Check sheet for the modelled part. Datum: model origin and axes. Units: mm. A direction names the side the tool comes from. Give positions to 0.01 mm unless a question says otherwise; leave off trailing zeros. Loops run counter-clockwise (first coordinate to the right, second up) from the corner with the lowest first, then second, coordinate; pieces in that order, holes last. Notation, with made-up numbers: M 66,-25.75 L 71,-25.75 A14 cw 71,1.25 Z; hole C 50.5,79 d9. An arc over 180 degrees is marked long. One line per question, with ' | ' between items. Start each with the question number.
Autodesk Inventor part; units mm, degrees
ref_plane "YZ Plane" through (0, 0, 0) normal (1, 0, 0) x (0, 1, 0)
ref_plane "XZ Plane" through (0, 0, 0) normal (0, 1, 0) x (-1, 0, 0)
sketch "Sketch1" plane through (0, 0, 0) normal (0, 0, 1) x (1, 0, 0)
  line L0 (0, 3.81) -> (1.746, 3.81)
  line L1 (0, 0) -> (0, 7.4896) construction
  line L2 (0, 0) -> (13.1944, 0) construction
  line L3 (0, -3.81) -> (1.746, -3.81)
  arc A0 (1.746, -3.81) -> (1.746, 3.81) centre (0, 0) ccw
  line L4 (0, 3.81) -> (0, -3.81)
  point P0 (-6.8886, 3.81)
  point P1 (6.6767, 3.81)
  point P2 (0, 4.191)
  point P3 (0, 4.191)
  point P4 (-6.8886, -3.81)
  point P5 (6.6767, -3.81)
  point P6 (0, 4.191)
  point P7 (4.191, 0)
  dimension "d1" = 0.381
  dimension "d11" = 4.191
revolve "Revolution1" add sketch "Sketch1" angle 360 about axis through (0, 0, 0) along (0, 1, 0)
sketch "Sketch2" plane through (0, 3.81, 0) normal (0, 1, 0) x (1, 0, 0)
  circle A0 centre (0, 0) radius 1.746
  dimension "d3" = 3.4919
hole "Hole1" at (0, 3.81, 0) direction (0, -1, 0) diameter 3.4798 end through all
ref_plane "Work Plane1" through (0, 0, 4.191) normal (0, 0, 1) x (1, 0, 0)
sketch "Sketch3" plane through (0, 0, 4.191) normal (0, 0, 1) x (1, 0, 0)
  line L0 (-2.159, 2.54) -> (2.159, 2.54)
  line L1 (2.159, 2.54) -> (2.159, -1.27)
  line L2 (2.159, -1.27) -> (-2.159, -1.27)
  line L3 (-2.159, -1.27) -> (-2.159, 2.54)
  line L4 (1.746, 3.81) -> (-1.746, 3.81)
  point P0 (0, 0)
  point P1 (0, 2.54)
  dimension "d13" = 4.318
  dimension "d14" = 3.81
  dimension "d15" = 1.27
extrude "Extrusion1" add sketch "Sketch3" along normal blind 10.16
ref_plane "Work Plane2" through (0, 0, 1.7399) normal (0, 0, 1) x (1, 0, 0)
extrude "Extrusion2" add sketch "Sketch3" against normal up to surface (2.4511 mm away)
sketch "Sketch4" plane through (0, -1.27, 0) normal (0, -1, 0) x (1, 0, 0)
  line L0 (2.159, 2.54) -> (2.159, 14.351)
  line L1 (2.159, 10.541) -> (-2.159, 10.541)
  line L2 (-2.159, 10.541) -> (-2.159, 14.351)
  line L3 (-2.159, 14.351) -> (2.159, 14.351)
  line L4 (2.159, 14.351) -> (2.159, 10.541) construction
  line L5 (-2.159, 14.351) -> (2.159, 14.351)
  circle A0 centre (0, 15.689) radius 0.635
  circle A1 centre (0, 15.689) radius 2.54
  circle A2 centre (-1.651, 18.401) radius 0.635
  circle A3 centre (-1.651, 18.401) radius 2.54
  point P0 (0, 0)
  point P1 (2.159, 14.351)
  point P2 (0, 14.351)
  point P3 (2.159, 14.351)
  point P4 (0.889, 18.401)
  point P5 (-2.5191, 16.014)
  point P6 (-1.3208, 17.8586)
  point P7 (0.8681, 18.0761)
  dimension "d31" = 5.08
  dimension "d22" = 3.81
  dimension "d25" = 1.27
  dimension "d27" = 5.08
  dimension "d30" = 1.27
  dimension "d32" = 1.27
  dimension "d33" = 4.318
extrude "Extrusion4" add sketch "Sketch4" along normal blind 1.27
properties part number "Left Arm" material "Phenolic Resin"
Q1. Depth check by flat-ended pin: P1, Ø1.5, axis at x = 0, z = 15.689, coming from the +Y side; P2, Ø1.5, axis at x = -1.651, z = 18.401, coming from the -Y side; P3, Ø4.5, axis at x = 0, z = 8, coming from the +Y side. Enter the tip coordinate at first touch or a pass-through.
Q2. Cross-section at B-B (y = -2). Record the cut outline in (x, z) (3 decimals).
Q3. Cross-section at D-D (y = -1). Record the cut outline in (x, z).
Q4. Material ranges on probe 1 along Z at (x, y) = (0, 1.75); probe 2 along Z at (x, y) = (0, -1.9); probe 3 along X at (y, z) = (0.25, 9.75), recorded low to high. Write a range as from..to.
Q5. Cross-section at C-C (x = 0). State how many separate pieces and enclosed holes the cut face has, and give its area (3 significant figures).
Q6. Draft check along Z on faces 4 (the flat face through (0, 1, 14.351)), 5 (the cylindrical face through (-3.039, -1.896, 20.528)), 6 (the flat face through (0, 2.54, 9)). Enter one of: released by +Z, released by -Z, zero draft, split by the parting line, or undercut.
Q7. Access from +Z, -Z, +X, -X, +Y, -Y to the whole of each face (thin tool, end or side, straight path). Record for faces 1 (the flat face through (0, -2, 10.541)), 2 (the flat face through (-1, -2.54, 16)), 3 (the flat face through (-0.9, -1.27, 17.7)).
Solved:
1) P1: stops at y = -1.27 | P2: stops at y = -2.54 | P3: stops at y = 2.54
2) outline: C 0,0 d7.366; M -2.519,16.014 A2.54 ccw -2.159,14.351 L -2.159,10.541 L 2.159,10.541 L 2.159,14.351 A2.54 ccw 0.868,18.076 A2.54 ccw long Z; hole C -1.651,18.401 d1.27; hole C 0,0 d3.48; hole C 0,15.689 d1.27
3) outline: M -2.16,3.45 A4.07 ccw long 2.16,3.45 L 2.16,14.35 L -2.16,14.35 Z; hole C 0,0 d3.48
4) probe 1: z = -3.81..-1.74, 1.74..14.35 | probe 2: z = -3.74..-1.74, 1.74..3.74, 10.54..15.05, 16.32..20.33 | probe 3: x = -2.16..2.16
5) separate pieces: 3 | enclosed holes: 0 | area: 77.2 mm²
6) face 4: released by +Z | face 5: undercut | face 6: zero draft
7) face 1: +X, -X, -Y | face 2: +Z, +X, -X, -Y | face 3: +Z, +X, -X, +Y
